Here's how the part is built. I have some questions about the finished solid (model axes, mm). Give positions to 0.01 mm unless a question says otherwise; leave off trailing zeros. Write each loop counter-clockwise with the first axis right and the second up, starting at its lowest first coordinate (ties: lowest second). Pieces come first, ordered by that corner, then holes. Notation, with made-up numbers: (74, 17.25) -> (130, 17.25) arc R20 cw to (130, 39.25) -> close; hole circle Ø2 at (78, -36). An arc over 180 degrees is marked (long way). Return JSON: item names as keys, results as strings.
from build123d import *

# Parameters (mm, degrees)
SKETCH1_W           = 40
SKETCH1_H           = 40
SKETCH1_R           = 9
SKETCH1_R_2         = 1.5
BOSS_EXTRUDE1_DEPTH = 5


with BuildPart() as part:
    # Sketch1 → Boss-Extrude1 (new body)
    with BuildSketch(Plane(origin=(0, 0, 0), x_dir=(0, 0, -1), z_dir=(1, 0, 0))):
        with Locations((33.747195152, -20)):
            Rectangle(SKETCH1_W, SKETCH1_H)
        with Locations((33.747195152, -28)):
            Circle(SKETCH1_R, mode=Mode.SUBTRACT)
        with Locations((18.685090131, -6.89933539)):
            Circle(SKETCH1_R_2, mode=Mode.SUBTRACT)
        with Locations(Location((18.685090131, -33.10066461, 0), (0, 0, 180))):
            Circle(SKETCH1_R_2, mode=Mode.SUBTRACT)
        with Locations((48.809300173, -33.10066461)):
            Circle(SKETCH1_R_2, mode=Mode.SUBTRACT)
        with Locations(Location((48.809300173, -6.89933539, 0), (0, 0, 180))):
            Circle(SKETCH1_R_2, mode=Mode.SUBTRACT)
    extrude(amount=BOSS_EXTRUDE1_DEPTH)


solid = part.part
1. If I drill on line 1 (Z direction, x = 3.3, y = -34); line 2 (Z direction, x = 0.45, y = -6.5); line 3 (Z direction, x = 3, y = -33.5), over which ranges is the centre line in solid material (lowest first)? Write a range as [from, to].
Taken from the geometry:
{"line 1": "z = [-53.75, -50.01], [-47.61, -40.46], [-27.04, -19.89], [-17.48, -13.75]", "line 2": "z = [-53.75, -50.26], [-47.36, -20.13], [-17.24, -13.75]", "line 3": "z = [-53.75, -50.26], [-47.36, -40.87], [-26.62, -20.13], [-17.24, -13.75]"}
2. If we mould it in two halves opening along Y, with no side actions, what happens to faces 1 (the face through (2, -20, -13.747)), 2 (the face through (2.465, -6.833, -17.187)), 3 (the face through (2.465, -34.365, -17.879)), 4 (the face through (2, 0, -33))? For each: released by +Y, released by -Y, zero draft, split by the parting line, or undercut.
Taken from the geometry:
{"face 1": "zero draft", "face 2": "undercut", "face 3": "undercut", "face 4": "released by +Y"}
3. Suppose I cut it at C-C, the plane x = 3.95. List the corners of the cut face in (y, z) for me.
Taken from the geometry:
{"outline": "(-40, -53.75) -> (0, -53.75) -> (0, -13.75) -> (-40, -13.75) -> close; hole circle Ø18 at (-28, -33.75); hole circle Ø3 at (-33.1, -48.81); hole circle Ø3 at (-33.1, -18.69); hole circle Ø3 at (-6.9, -48.81); hole circle Ø3 at (-6.9, -18.69)"}
4. Suppose I cut it at B-B, the plane z = -28.5. List the corners of the cut face in (x, y) for me.
Taken from the geometry:
{"outline": "(0, -40) -> (5, -40) -> (5, -35.31) -> (0, -35.31) -> close; (0, -20.69) -> (5, -20.69) -> (5, 0) -> (0, 0) -> close"}
5. Suppose I cut it at A-A, the plane y = -28. List the corners of the cut face in (x, z) for me, and give its area (3 significant figures).
Taken from the geometry:
{"outline": "(0, -53.75) -> (5, -53.75) -> (5, -42.75) -> (0, -42.75) -> close; (0, -24.75) -> (5, -24.75) -> (5, -13.75) -> (0, -13.75) -> close", "area": "110 mm²"}
6. For pin 1 Ø1.8 at (y, z) = (-33.1, -18.69) entering from -X, with a flat end and sliding along its axis, tell me the tip position at first contact or that it passes through.
Taken from the geometry:
{"pin 1": "passes through"}
